```python
from build123d import *

# Parameters (mm, degrees)
SKETCH1_R      = 8.5
EXTRUDE1_DEPTH = 1
EXTRUDE2_DEPTH = 4
SKETCH3_R      = 6.8
EXTRUDE3_DEPTH = 10


with BuildPart() as part:
    # Sketch1 → Extrude1 (new body)
    with BuildSketch(Plane(origin=(0, 0, 0), x_dir=(1, 0, 0), z_dir=(0, 1, 0))):
        with Locations(Location((0, 0, 0), (0, 0, 270))):
            Circle(SKETCH1_R)
    extrude(amount=EXTRUDE1_DEPTH)

    # Sketch2 → Extrude2 (add)
    with BuildSketch(Plane(origin=(0, 1, 0), x_dir=(1, 0, 0), z_dir=(0, 1, 0))):
        Polygon((0, 8.5), (-7.361215932, 4.25), (-7.361215932, -4.25), (0, -8.5), (7.361215932, -4.25), (7.361215932, 4.25), align=None)
    extrude(amount=EXTRUDE2_DEPTH)

    # Sketch3 → Extrude3 (add)
    with BuildSketch(Plane.XZ):
        with Locations(Location((0, 0, 0), (0, 0, 90))):
            Circle(SKETCH3_R)
    extrude(amount=EXTRUDE3_DEPTH)


solid = part.part
```
For this review, take the finished solid that the model builds, in its own axes (mm). A direction names the side the tool comes from. Coordinates: 2 decimals unless noted, no trailing zeros. Loops run counter-clockwise (first coordinate to the right, second up) from the corner with the lowest first, then second, coordinate; pieces in that order, holes last.
1. Add section D-D, the plane y = 0.5. Give the boundary of the cut face in (x, z).
2. Insertion check: P1, Ø1, axis at x = -3.5, y = -7, coming from the -Z side; P2, Ø0.9, axis at x = -8, z = 2, coming from the +Y side; P3, Ø1.2, axis at y = 3, z = -1, coming from the +X side. Each pin has a flat end and moves straight along its axis. Give the tip position at first contact, or say it passes through.
3. Add section B-B, the plane x = -4.5. Give the boundary of the cut face in (y, z).
4. For line 1 (X direction, y = 1.75, z = -2.25); line 2 (Y direction, x = 5.5, z = 4.5); line 3 (Y direction, x = 6.25, z = -5.5), list the stretches that pass through material, from the lowest coordinate up.
5. For faces 1 (the flat face through (3.732, 2.972, -6.345)), 2 (the cylindrical face through (6.64, -4.93, -1.47)), 3 (the flat face through (-3.732, 2.972, 6.345)), 4 (the flat face through (3.629, 2.972, 6.405)), 5 (the flat face through (8, 1, 0)), list the 3-axis set-ups (+Z, -Z, +X, -X, +Y, -Y) from which the entire face can be reached by the end or side of a thin tool; tool diameter is ignored.
6. Add section A-A, the plane y = 2.75. Give the boundary of the cut face in (x, z).
7. Add section C-C, the plane z = 0. Give the boundary of the cut face in (x, y), then the cut area to 3 significant figures.
Result:
1. outline: circle Ø17 at (0, 0)
2. P1: stops at z = -6.1
2. P2: stops at y = 1
2. P3: stops at x = 7.36
3. outline: (-10, -5.1) - (0, -5.1) - (0, -7.21) - (1, -7.21) - (1, -5.9) - (5, -5.9) - (5, 5.9) - (1, 5.9) - (1, 7.21) - (0, 7.21) - (0, 5.1) - (-10, 5.1) - close
4. line 1: x = -7.36 to 7.36
4. line 2: y = 0 to 5
4. line 3: y = 0 to 1
5. face 1: -Z, +X, +Y
5. face 2: -Y
5. face 3: +Z, -X, +Y
5. face 4: +Z, +X, +Y
5. face 5: +Z, -Z, +X, +Y
6. outline: (-7.36, -4.25) - (0, -8.5) - (7.36, -4.25) - (7.36, 4.25) - (0, 8.5) - (-7.36, 4.25) - close
7. outline: (-8.5, 0) - (-6.8, 0) - (-6.8, -10) - (6.8, -10) - (6.8, 0) - (8.5, 0) - (8.5, 1) - (7.36, 1) - (7.36, 5) - (-7.36, 5) - (-7.36, 1) - (-8.5, 1) - close
7. area: 212 mm2
